Check sheet for the modelled part. Datum: model origin and axes. Units: mm. Give positions to 0.01 mm unless a question says otherwise; leave off trailing zeros. Loops run counter-clockwise (first coordinate to the right, second up) from the corner with the lowest first, then second, coordinate; pieces in that order, holes last. Notation, with made-up numbers: M 7.25,10.25 L 44.25,10.25 A21 cw 44.25,49.25 Z; hole C 89.25,-2.75 d8. An arc over 180 degrees is marked long. Write each question's results on one line, items separated by ' | '. Start each with the question number.
1. Material ranges on line 1 along X through (y, z) = (-4.5, 106); line 2 along X through (y, z) = (-9.75, 57); line 3 along X through (y, z) = (-6.5, 81), recorded low to high.
2. Sectioned sample at B-B on y = -10.25. Record the cut outline in (x, z), and give its area (3 significant figures).
3. Sectioned sample at A-A on x = 819. Record the cut outline in (y, z), and give its area (3 significant figures).
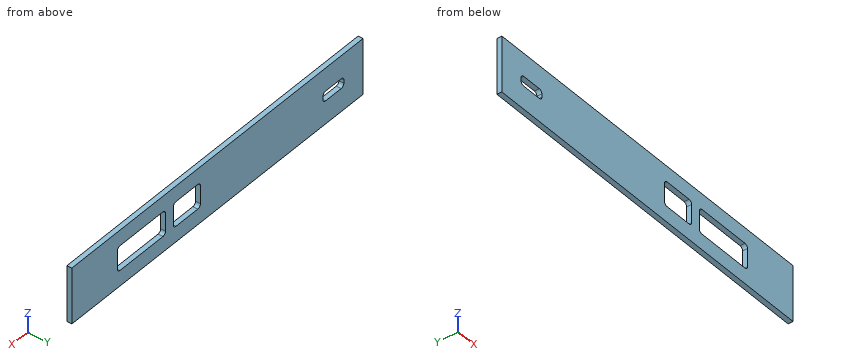
```python
from build123d import *

# Parameters (mm, degrees)
SKETCH_W     = 1119
SKETCH_H     = 172
PAD_DEPTH    = 15
POCKET_DEPTH = 15.001


with BuildPart() as part:
    # Sketch → Pad (new body)
    with BuildSketch(Plane.XZ):
        with Locations((559.5, 86)):
            Rectangle(SKETCH_W, SKETCH_H)
    extrude(amount=PAD_DEPTH)

    # Sketch001 (on Face6 of Pad) → Pocket (cut, through all)
    with BuildSketch(Plane.XZ.offset(15)):
        with BuildLine():
            ThreePointArc((635, 124), (627.928932, 121.071068), (625, 114))
            Line((625, 58), (625, 114))
            ThreePointArc((625, 58), (627.928932, 50.928932), (635, 48))
            Line((719, 48), (635, 48))
            ThreePointArc((719, 48), (726.071068, 50.928932), (729, 58))
            Line((729, 114), (729, 58))
            ThreePointArc((729, 114), (726.071068, 121.071068), (719, 124))
            Line((635, 124), (719, 124))
        make_face()
        with BuildLine():
            ThreePointArc((769, 124), (761.928932, 121.071068), (759, 114))
            Line((759, 58), (759, 114))
            ThreePointArc((759, 58), (761.928932, 50.928932), (769, 48))
            Line((934, 48), (769, 48))
            ThreePointArc((934, 48), (941.071068, 50.928932), (944, 58))
            Line((944, 114), (944, 58))
            ThreePointArc((944, 114), (941.071068, 121.071068), (934, 124))
            Line((769, 124), (934, 124))
        make_face()
        with BuildLine():
            ThreePointArc((84, 101), (76.928932, 98.071068), (74, 91))
            Line((74, 81), (74, 91))
            ThreePointArc((74, 81), (76.928932, 73.928932), (84, 71))
            Line((144, 71), (84, 71))
            ThreePointArc((144, 71), (151.071068, 73.928932), (154, 81))
            Line((154, 91), (154, 81))
            ThreePointArc((154, 91), (151.071068, 98.071068), (144, 101))
            Line((84, 101), (144, 101))
        make_face()
    extrude(amount=-POCKET_DEPTH, mode=Mode.SUBTRACT)


solid = part.part
```
Output values:
1) line 1: 0 to 625, 729 to 759, 944 to 1119 | line 2: 0 to 625.05, 728.95 to 759.05, 943.95 to 1119 | line 3: 0 to 74, 154 to 625, 729 to 759, 944 to 1119
2) outline: M 0,0 L 1119,0 L 1119,172 L 0,172 Z; hole M 74,81 A10 ccw 84,71 L 144,71 A10 ccw 154,81 L 154,91 A10 ccw 144,101 L 84,101 A10 ccw 74,91 Z; hole M 625,58 A10 ccw 635,48 L 719,48 A10 ccw 729,58 L 729,114 A10 ccw 719,124 L 635,124 A10 ccw 625,114 Z; hole M 759,58 A10 ccw 769,48 L 934,48 A10 ccw 944,58 L 944,114 A10 ccw 934,124 L 769,124 A10 ccw 759,114 Z | area: 168,000 mm2
3) outline: M -15,0 L 0,0 L 0,48 L -15,48 Z; M -15,124 L 0,124 L 0,172 L -15,172 Z | area: 1,440 mm2
